The listing builds one solid part. Answer for the finished solid, in the listing's coordinates (mm). A direction names the side the tool comes from. Round coordinates to 2 decimals unless told otherwise and drop trailing zeros. Write each loop counter-clockwise with the first axis right and the second up, starting at its lowest first coordinate (ties: lowest second). Pieces come first, ordered by that corner, then holes. Notation, with made-up numbers: (40.5, -24) - (47.5, -24) arc R28 cw to (47.5, 4) - close; hole circle Ø6 at (89.25, 62). An arc over 180 degrees is marked (long way). Answer as CSV lines item,"result". Start each with the question number.
Item 1: Which of the six approach directions +Z, -Z, +X, -X, +Y, -Y give full straight-line access (tool end or side, diameter ignored) to faces 5 (the flat face through (0, 126, -5.5)), 6 (the flat face through (7.5, 122, 0))?
Item 2: A flat-ended cylindrical pin translates along its axis: pin 1 (2.5 mm diameter, centred on y = 20, z = 0, fed in from +X). Find the tip coordinate at first contact, or state that the pin passes through.
Item 3: Straight lines are drawn through the part: line 1 along Y through (x, z) = (6.5, 0); line 2 along Z through (x, y) = (-2.5, 207). For each, find the intervals that lie inside material, in ascending order. Write a range as [from, to].
Item 4: For a pull along X with two mould halves and no side action, classify faces 1 (the flat face through (-7, 248, 0)), 2 (the flat face through (5.5, 126, 0)), 3 (the flat face through (-7.5, 122, 0)), 4 (the flat face through (-5.5, 126, 0)) as pulls with the +X half, pulls with the -X half, needs draft (parallel to the pull), parting line crosses it, or undercut.
Item 5: A cutting plane is placed at B-B on y = 166. Determine the outline of the cut face in (x, z), and give its area (3 significant figures).
Item 6: A cutting plane is placed at A-A on y = 208. Determine the outline of the cut face in (x, z), and give its area (3 significant figures).
```python
from build123d import *

# Parameters (mm, degrees)
SKETCH_1_W          = 15
SKETCH_1_H          = 15
EXTRUDE_1_DEPTH     = 248
SKETCH_3_R          = 1.5
CUT_EXTRUDE_2_DEPTH = 15
CUT_EXTRUDE_3_DEPTH = 15
SKETCH_5_W          = 11
SKETCH_5_H          = 11
CUT_EXTRUDE_4_DEPTH = 248
SKETCH_6_R          = 2.5
CUT_EXTRUDE_5_DEPTH = 15


with BuildPart() as part:
    # 草图1 → 凸台-拉伸1 (new body)
    with BuildSketch(Plane(origin=(0, 0, 0), x_dir=(1, 0, 0), z_dir=(0, 1, 0))):
        Rectangle(SKETCH_1_W, SKETCH_1_H)
    extrude(amount=EXTRUDE_1_DEPTH)

    # 草图3 → 切除-拉伸2 (cut)
    with BuildSketch(Plane(origin=(7.5, 0, 0), x_dir=(0, 0, -1), z_dir=(1, 0, 0))):
        with Locations((0, 5)):
            Circle(SKETCH_3_R)
        with Locations((0, 20)):
            Circle(SKETCH_3_R)
    extrude(amount=-CUT_EXTRUDE_2_DEPTH, mode=Mode.SUBTRACT)

    # 草图4 → 切除-拉伸3 (cut)
    with BuildSketch(Plane.XY.offset(7.5)):
        with BuildLine():
            Line((-1.5, 70), (-1.5, 80))
            ThreePointArc((-1.5, 80), (0, 81.5), (1.5, 80))
            Line((1.5, 80), (1.5, 70))
            ThreePointArc((1.5, 70), (0, 68.5), (-1.5, 70))
        make_face()
    extrude(amount=-CUT_EXTRUDE_3_DEPTH, mode=Mode.SUBTRACT)

    # 草图5 → 切除-拉伸4 (cut)
    with BuildSketch(Plane(origin=(0, 248, 0), x_dir=(1, 0, 0), z_dir=(0, 1, 0))):
        Rectangle(SKETCH_5_W, SKETCH_5_H)
    extrude(amount=-CUT_EXTRUDE_4_DEPTH, mode=Mode.SUBTRACT)

    # 草图6 → 切除-拉伸5 (cut)
    with BuildSketch(Plane.ZY.offset(7.5)):
        with Locations((0, 208)):
            Circle(SKETCH_6_R)
        with Locations((0, 178)):
            Circle(SKETCH_6_R)
    extrude(amount=-CUT_EXTRUDE_5_DEPTH, mode=Mode.SUBTRACT)


solid = part.part
```
Geometry says:
1,face 5,"+Y, -Y"
1,face 6,"+Z, -Z, +X, +Y, -Y"
2,pin 1,"passes through"
3,line 1,"y = [0, 3.5], [6.5, 18.5], [21.5, 175.5], [180.5, 205.5], [210.5, 248]"
3,line 2,"z = [-7.5, -5.5], [5.5, 7.5]"
4,face 1,"needs draft"
4,face 2,"undercut"
4,face 3,"pulls with the -X half"
4,face 4,"undercut"
5,outline,"(-7.5, -7.5) - (7.5, -7.5) - (7.5, 7.5) - (-7.5, 7.5) - close; hole (-5.5, -5.5) - (5.5, -5.5) - (5.5, 5.5) - (-5.5, 5.5) - close"
5,area,"104 mm^2"
6,outline,"(-7.5, -7.5) - (7.5, -7.5) - (7.5, -2.5) - (5.5, -2.5) - (5.5, -5.5) - (-5.5, -5.5) - (-5.5, -2.5) - (-7.5, -2.5) - close; (-7.5, 2.5) - (-5.5, 2.5) - (-5.5, 5.5) - (5.5, 5.5) - (5.5, 2.5) - (7.5, 2.5) - (7.5, 7.5) - (-7.5, 7.5) - close"
6,area,"84.0 mm^2"
